from build123d import *

# Parameters (mm, degrees)
F0_R     = 7
F1_DEPTH = 50
F3_R     = 3
F4_DEPTH = 25
F5_R     = 1.5


with BuildPart() as f1:
    # F0 (on Front) → F1 (new body)
    with BuildSketch(Plane.XZ):
        with BuildLine():
            Line((2, -30), (2, -7.7459666924))
            ThreePointArc((2, -7.7459666924), (0, 8), (-2, -7.7459666924))
            Line((-2, -7.7459666924), (-2, -30))
            Line((-2, -30), (0, -30))
            Line((0, -30), (2, -30))
        make_face()
        Circle(F0_R, mode=Mode.SUBTRACT)
    extrude(amount=F1_DEPTH)

    # F3 (on face) → F4 (cut)
    with BuildSketch(Plane(origin=(-2, 0, 0), x_dir=(0, -1, 0), z_dir=(-1, 0, 0))):
        Polygon((50, -7.7459666924), (34, -7.7459666924), (23, -30), (50, -30), align=None)
        Polygon((8, -30), (0, -7.7459666924), (0, -30), align=None)
        with Locations((16, -25)):
            Circle(F3_R)
    extrude(amount=-F4_DEPTH, mode=Mode.SUBTRACT)

    # F5 (call 1 of 2: OpenCascade refuses the feature's edges together)
    f5_edges = [f1.edges().sort_by_distance(p)[0] for p in [
        (-2, -17, -7.745967),
    ]]
    fillet(f5_edges, radius=F5_R)

    # F5#2 (call 2 of 2)
    f5_2_edges = [f1.edges().sort_by_distance(p)[0] for p in [
        (2, -17, -7.745967),
    ]]
    fillet(f5_2_edges, radius=F5_R)


solid = f1.part
Input: part model. Units: mm. Frame: model coordinates. A direction names the side the tool comes from. Give positions to 0.01 mm unless a question says otherwise; leave off trailing zeros. Write each loop counter-clockwise with the first axis right and the second up, starting at its lowest first coordinate (ties: lowest second). Pieces come first, ordered by that corner, then holes.
Q1. Section D-D, the plane y = -9.5. Output: boundary loops of the cut face in (x, z), plus the area to 3 significant figures.
Q2. Set-up query: faces 1 (the face through (0, -13.6, -26.8)), 2 (the face through (-0.035, -4.056, -19.029)), 3 (the face through (-2, -17, -17)), 4 (the face through (0, -42, -7.746)), 5 (the face through (2, -17, -17)). Return all of +Z, -Z, +X, -X, +Y, -Y with unobstructed straight access to the full face (end or side cutting, diameter ignored); none if empty.
Q3. Material intervals for probe 1 along Z at (x, y) = (0, -14); probe 2 along Z at (x, y) = (0.85, -16); probe 3 along Z at (x, y) = (-6.25, -28), sorted ascending.
Q4. Section A-A, the plane y = -16. Output: boundary loops of the cut face in (x, z).
Q5. Section B-B, the plane x = 0.5. Output: boundary loops of the cut face in (y, z), plus the area to 3 significant figures.
Q6. Pull-direction query (Z, two-part tool) for faces 6 (the face through (6.466, -24.65, -2.681)), 7 (the face through (4, 0, -6)), 8 (the face through (0, -15, -30)); classes: pulls with the +Z half, pulls with the -Z half, needs draft (parallel to the pull), parting line crosses it, or undercut.
Q7. Section C-C, the plane z = -25. Output: boundary loops of the cut face in (x, y), plus the area to 3 significant figures.
Q8. First-contact query: P1, Ø8, axis at y = -11, z = -9.5, coming from the -X side; P2, Ø2, axis at x = 1, y = -41, coming from the -Z side; P3, Ø17, axis at y = -22.5, z = -16.5, coming from the +X side. Flat tips, straight axial feed; report the tip coordinate or a pass-through.
Filled in:
1. outline: (-2.95, -7.44) arc R1.5 cw to (-2, -8.83) - (-2, -30) - (2, -30) - (2, -8.83) arc R1.5 cw to (2.95, -7.44) arc R8 ccw (long way) to start; hole circle Ø14 at (0, 0)
1. area: 136 mm2
2. face 1: +X, -X
2. face 2: -Z, +X, -X, +Y
2. face 3: -Z, -X, +Y, -Y
2. face 4: -Z, +X, -X, -Y
2. face 5: -Z, +X, +Y, -Y
3. probe 1: z = -30 to -27.24, -22.76 to -7, 7 to 8
3. probe 2: z = -30 to -28, -22 to -6.95, 6.95 to 7.95
3. probe 3: z = -4.99 to -3.15, 3.15 to 4.99
4. outline: (-2.95, -7.44) arc R1.5 cw to (-2, -8.83) - (-2, -22) - (2, -22) - (2, -8.83) arc R1.5 cw to (2.95, -7.44) arc R8 ccw (long way) to start; (-2, -30) - (2, -30) - (2, -28) - (-2, -28) - close; hole circle Ø14 at (0, 0)
5. outline: (-50, -7.75) - (-34, -7.75) - (-23, -30) - (-8, -30) - (0, -7.75) - (0, -6.98) - (-50, -6.98) - close; (-50, 6.98) - (0, 6.98) - (0, 7.98) - (-50, 7.98) - close; hole circle Ø6 at (-16, -25)
5. area: 605 mm2
6. face 6: undercut
6. face 7: needs draft
6. face 8: pulls with the -Z half
7. outline: (-2, -25.47) - (2, -25.47) - (2, -19) - (-2, -19) - close; (-2, -13) - (2, -13) - (2, -6.2) - (-2, -6.2) - close
7. area: 53.1 mm2
8. P1: stops at x = -5.81
8. P2: stops at z = -7.75
8. P3: stops at x = 2.25
